from build123d import *

# Parameters (mm, degrees)
SKETCH1_W                           = 203.2
SKETCH1_H                           = 63.5
BOSS_EXTRUDE1_DEPTH                 = 3.175
F_9_32_0_28125_DIAMETER_HOLE1_D     = 7.14375
F_9_32_0_28125_DIAMETER_SLOT1_DEPTH = 3.175
FILLET1_R                           = 3.175


# Read off the part's stored shape, not the designer's step: 9/32 (0.28125) Diameter Slot1
with BuildPart() as part:
    # Sketch1 → Boss-Extrude1 (new body)
    with BuildSketch(Plane(origin=(0, 0, 0), x_dir=(1, 0, 0), z_dir=(0, 1, 0))):
        with Locations((101.6, 31.75)):
            Rectangle(SKETCH1_W, SKETCH1_H)
    extrude(amount=BOSS_EXTRUDE1_DEPTH)

    # 9/32 (0.28125) Diameter Hole1 (through all)
    with Locations(Plane(origin=(0, 3.175, 0), x_dir=(1, 0, 0), z_dir=(0, 1, 0))):
        with Locations((12.7, 12.7), (12.7, 50.8), (88.9, 31.75)):
            Hole(F_9_32_0_28125_DIAMETER_HOLE1_D / 2)

    # 9/32 (0.28125) Diameter Slot1 outline → 9/32 (0.28125) Diameter Slot1 (cut)
    with BuildSketch(Plane(origin=(0, 0, 0), x_dir=(1, 0, 0), z_dir=(0, 1, 0))):
        with BuildLine():
            Line((187.721875, 9.128125), (193.278125, 9.128125))
            ThreePointArc((193.278125, 9.128125), (196.85, 12.7), (193.278125, 16.271875))
            Line((193.278125, 16.271875), (187.721875, 16.271875))
            ThreePointArc((187.721875, 16.271875), (184.15, 12.7), (187.721875, 9.128125))
        make_face()
        with BuildLine():
            Line((187.721875, 47.228125), (193.278125, 47.228125))
            ThreePointArc((193.278125, 47.228125), (196.85, 50.8), (193.278125, 54.371875))
            Line((193.278125, 54.371875), (187.721875, 54.371875))
            ThreePointArc((187.721875, 54.371875), (184.15, 50.8), (187.721875, 47.228125))
        make_face()
        with BuildLine():
            Line((111.521875, 28.178125), (117.078125, 28.178125))
            ThreePointArc((117.078125, 28.178125), (120.65, 31.75), (117.078125, 35.321875))
            Line((117.078125, 35.321875), (111.521875, 35.321875))
            ThreePointArc((111.521875, 35.321875), (107.95, 31.75), (111.521875, 28.178125))
        make_face()
    extrude(amount=F_9_32_0_28125_DIAMETER_SLOT1_DEPTH, mode=Mode.SUBTRACT)

    # Fillet1
    fillet1_edges = [part.edges().sort_by_distance(p)[0] for p in [
        (0, 1.5875, -63.5),
        (203.2, 1.5875, -63.5),
        (203.2, 1.5875, 0),
        (0, 1.5875, 0),
    ]]
    fillet(fillet1_edges, radius=FILLET1_R)


solid = part.part
Build history of the part. All positions in model axes, mm. A direction names the side the tool comes from. Coordinates: 2 decimals unless noted, no trailing zeros. Order: outer loops, then holes, each group sorted by start corner. A loop starts at its lowest first (then second) coordinate and runs counter-clockwise, first axis right, second up. Notation, with made-up numbers: M 84,54.5 L 142,54.5 A21 ccw 142,78.5 Z; hole C -15.5,-2 d1. An arc over 180 degrees is marked long. One line per question, with ' | ' between items. Start each with the question number.
Q1. Probe L1, parallel to X at y = 1, z = -31.75; L2, parallel to X at y = 1.25, z = -12.7; L3, parallel to Z at x = 12.7, y = 2.1. List the from-to ranges inside material, lowest first. Write a range as from..to.
Q2. Flat gauge pin, fed straight in: pin 1 Ø4.5 at (x, z) = (12.7, -50.8) entering from +Y. Where does the tip first touch, or does it go through?
Q3. Saw through at C-C (y = 1.6). List the corners of the cut face in (x, z) (3 decimals).
Q4. Saw through at A-A (x = 88.9). List the corners of the cut face in (y, z) (3 decimals).
Q5. Saw through at D-D (x = 12.7). List the corners of the cut face in (y, z) (3 decimals).
Q6. 3-axis set-ups, long thin cutter, end or side, ignore diameter. For faces 1 (the face through (100, 3.175, -32)), 2 (the face through (107.95, 1.57, -31.83)): which of +Z, -Z, +X, -X, +Y, -Y reach the whole face in a straight line?
Q7. Two-plate mould, pull along X, no slides. Class faces 3 (the face through (196.85, 1.57, -50.72)), 4 (the face through (100, 0, -32)): +X half, -X half, draft (parallel to the pull), parting line (faces both ways), or undercut.
Q8. Saw through at B-B (z = -50.8). List the corners of the cut face in (x, y) (3 decimals), then the cut area to 3 significant figures.
Check values:
1) L1: x = 0..85.33, 92.47..107.95, 120.65..203.2 | L2: x = 0..9.13, 16.27..184.15, 196.85..203.2 | L3: z = -63.5..-54.37, -47.23..-16.27, -9.13..0
2) pin 1: passes through
3) outline: M 0,-60.325 A3.175 ccw 3.175,-63.5 L 200.025,-63.5 A3.175 ccw 203.2,-60.325 L 203.2,-3.175 A3.175 ccw 200.025,0 L 3.175,0 A3.175 ccw 0,-3.175 Z; hole C 12.7,-50.8 d7.144; hole C 12.7,-12.7 d7.144; hole C 88.9,-31.75 d7.144; hole M 111.522,-35.322 L 117.078,-35.322 A3.572 ccw 117.078,-28.178 L 111.522,-28.178 A3.572 ccw Z; hole M 187.722,-54.372 L 193.278,-54.372 A3.572 ccw 193.278,-47.228 L 187.722,-47.228 A3.572 ccw Z; hole M 187.722,-16.272 L 193.278,-16.272 A3.572 ccw 193.278,-9.128 L 187.722,-9.128 A3.572 ccw Z
4) outline: M 0,-63.5 L 3.175,-63.5 L 3.175,-35.322 L 0,-35.322 Z; M 0,-28.178 L 3.175,-28.178 L 3.175,0 L 0,0 Z
5) outline: M 0,-63.5 L 3.175,-63.5 L 3.175,-54.372 L 0,-54.372 Z; M 0,-47.228 L 3.175,-47.228 L 3.175,-16.272 L 0,-16.272 Z; M 0,-9.128 L 3.175,-9.128 L 3.175,0 L 0,0 Z
6) face 1: +Z, -Z, +X, -X, +Y | face 2: +Y, -Y
7) face 3: undercut | face 4: draft
8) outline: M 0,0 L 9.128,0 L 9.128,3.175 L 0,3.175 Z; M 16.272,0 L 184.15,0 L 184.15,3.175 L 16.272,3.175 Z; M 196.85,0 L 203.2,0 L 203.2,3.175 L 196.85,3.175 Z | area: 582 mm2
